```python
from build123d import *

# Parameters (mm, degrees)
BOSS_EXTRUDE1_DEPTH      = 2
BOSS_EXTRUDE1_DEPTH_BACK = 3
SKETCH1_R                = 16
SKETCH1_R_2              = 1.75
SKETCH1_R_3              = 1.25
SKETCH2_R                = 4.95
SKETCH2_R_2              = 2.95
BOSS_EXTRUDE3_DEPTH      = 3
SKETCH5_R                = 3.5
CUT_EXTRUDE2_DEPTH       = 4
SKETCH6_R                = 18
SKETCH6_R_2              = 16
BOSS_EXTRUDE4_DEPTH      = 5
CUT_EXTRUDE3_DEPTH       = 10
CUT_EXTRUDE3_DEPTH_BACK  = 3
SKETCH7_R                = 11
SKETCH8_R                = 5
CUT_EXTRUDE4_DEPTH       = 3


with BuildPart() as part:
    # Sketch1 → Boss-Extrude1 (new, two sides: drawn at the far end of the back side and taken through both)
    with BuildSketch(Plane(origin=(0, 0, 0), x_dir=(1, 0, 0), z_dir=(0, 1, 0)).offset(-BOSS_EXTRUDE1_DEPTH_BACK)):
        with Locations(Location((0, 0, 0), (0, 0, 270))):
            Circle(SKETCH1_R)
        with Locations(Location((0, 0, 0), (0, 0, 270))):
            Circle(SKETCH1_R_2, mode=Mode.SUBTRACT)
        with Locations(Location((-13.5, 0, 0), (0, 0, 270))):
            Circle(SKETCH1_R_3, mode=Mode.SUBTRACT)
        with Locations(Location((-4.171729424, 12.83926297, 0), (0, 0, 270))):
            Circle(SKETCH1_R_3, mode=Mode.SUBTRACT)
        with Locations(Location((10.921729424, 7.935100906, 0), (0, 0, 270))):
            Circle(SKETCH1_R_3, mode=Mode.SUBTRACT)
        with Locations(Location((10.921729424, -7.935100906, 0), (0, 0, 270))):
            Circle(SKETCH1_R_3, mode=Mode.SUBTRACT)
        with Locations(Location((-4.171729424, -12.83926297, 0), (0, 0, 270))):
            Circle(SKETCH1_R_3, mode=Mode.SUBTRACT)
    extrude(amount=BOSS_EXTRUDE1_DEPTH + BOSS_EXTRUDE1_DEPTH_BACK)

    # Sketch2 → Boss-Extrude3 (add)
    with BuildSketch(Plane(origin=(0, 2, 0), x_dir=(1, 0, 0), z_dir=(0, 1, 0))):
        with Locations(Location((0, 0, 0), (0, 0, 270))):
            Circle(SKETCH2_R)
        with Locations(Location((0, 0, 0), (0, 0, 270))):
            Circle(SKETCH2_R_2, mode=Mode.SUBTRACT)
    extrude(amount=BOSS_EXTRUDE3_DEPTH)

    # Sketch5 → Cut-Extrude2 (cut)
    with BuildSketch(Plane.XZ.offset(3)):
        with Locations(Location((0, 0, 0), (0, 0, 270))):
            Circle(SKETCH5_R)
    extrude(amount=-CUT_EXTRUDE2_DEPTH, mode=Mode.SUBTRACT)

    # Sketch6 → Boss-Extrude4 (add)
    with BuildSketch(Plane(origin=(0, 2, 0), x_dir=(1, 0, 0), z_dir=(0, 1, 0))):
        with Locations(Location((0, 0, 0), (0, 0, 270))):
            Circle(SKETCH6_R)
        Circle(SKETCH6_R_2, mode=Mode.SUBTRACT)
    extrude(amount=-BOSS_EXTRUDE4_DEPTH)

    # Sketch7 → Cut-Extrude3 (cut, two sides: drawn at the far end of the back side and taken through both)
    with BuildSketch(Plane(origin=(0, 2, 0), x_dir=(1, 0, 0), z_dir=(0, 1, 0)).offset(-CUT_EXTRUDE3_DEPTH_BACK)):
        with Locations(Location((0, 0, 0), (0, 0, 270))):
            Circle(SKETCH7_R)
    extrude(amount=CUT_EXTRUDE3_DEPTH + CUT_EXTRUDE3_DEPTH_BACK, mode=Mode.SUBTRACT)

    # Sketch8 → Cut-Extrude4 (cut)
    with BuildSketch(Plane(origin=(0, -1, 0), x_dir=(1, 0, 0), z_dir=(0, 1, 0))):
        with Locations(Location((0, 0, 0), (0, 0, 270))):
            Circle(SKETCH8_R)
    extrude(amount=-CUT_EXTRUDE4_DEPTH, mode=Mode.SUBTRACT)


solid = part.part
```
Model file for the job. Use its own axes, mm. A direction names the side the tool comes from. Coordinates: 2 decimals unless noted, no trailing zeros. Order: outer loops, then holes, each group sorted by start corner. A loop starts at its lowest first (then second) coordinate and runs counter-clockwise, first axis right, second up. Notation, with made-up numbers: (18.25, -2) -> (29.25, -2) arc R9 ccw to (29.25, 5) -> close; hole circle Ø11 at (35.25, -29.5). An arc over 180 degrees is marked (long way). Return JSON: item names as keys, results as strings.
Item 1: Slice it at B-B (z = 0). Write the cut outline in (x, y).
Model answer:
{"outline": "(-18, -3) -> (-14.75, -3) -> (-14.75, 2) -> (-18, 2) -> close; (-12.25, -3) -> (-5, -3) -> (-5, -1) -> (-11, -1) -> (-11, 2) -> (-12.25, 2) -> close; (5, -3) -> (18, -3) -> (18, 2) -> (11, 2) -> (11, -1) -> (5, -1) -> close"}
Item 2: Slice it at C-C (x = 10.5). Write the cut outline in (y, z).
Model answer:
{"outline": "(-3, -14.62) -> (2, -14.62) -> (2, -9.11) -> (-3, -9.11) -> close; (-3, -6.76) -> (2, -6.76) -> (2, -3.28) -> (-1, -3.28) -> (-1, 3.28) -> (2, 3.28) -> (2, 6.76) -> (-3, 6.76) -> close; (-3, 9.11) -> (2, 9.11) -> (2, 14.62) -> (-3, 14.62) -> close"}
Item 3: 3-axis set-ups, long thin cutter, end or side, ignore diameter. For faces 1 (the face through (-10.74, 0.48, -2.38)), 2 (the face through (10.161, -0.535, -8.927)): which of +Z, -Z, +X, -X, +Y, -Y reach the whole face in a straight line?
Model answer:
{"face 1": "+Y", "face 2": "+Y, -Y"}
Item 4: Mould opens along X. For faces 3 (the face through (10.161, -0.535, 6.943)), 4 (the face through (5.407, -0.465, 17.169)), 5 (the face through (-4.65, -0.535, 13.994)), 6 (the face through (8, 2, 8)) say: pulls with the +X half, pulls with the -X half, needs draft (parallel to the pull), parting line crosses it, or undercut.
Model answer:
{"face 3": "undercut", "face 4": "parting line crosses it", "face 5": "undercut", "face 6": "needs draft"}
Item 5: Slice it at D-D (y = 1). Write the cut outline in (x, z).
Model answer:
{"outline": "circle Ø36 at (0, 0); hole circle Ø2.5 at (-13.5, 0); hole circle Ø22 at (0, 0); hole circle Ø2.5 at (-4.17, -12.84); hole circle Ø2.5 at (-4.17, 12.84); hole circle Ø2.5 at (10.92, -7.94); hole circle Ø2.5 at (10.92, 7.94)"}
Item 6: Wall check: line 1 along X through (y, z) = (0.45, 0); line 2 along X through (y, z) = (0.45, -7); line 3 along Z through (x, y) = (12, -1.6). Give the ranges that are in metal, low to high. Write a range as from..to.
Model answer:
{"line 1": "x = -18..-14.75, -12.25..-11, 11..18", "line 2": "x = -16.58..-8.49, 8.49..10.09, 11.75..16.58", "line 3": "z = -13.42..-8.57, -7.3..7.3, 8.57..13.42"}
Item 7: Pin check, flat tips, straight feed: P1, Ø2, axis at x = -4.17, z = -12.84, coming from the +Y side; P2, Ø3, axis at y = -0.5, z = -7.5, coming from the +X side; P3, Ø2, axis at x = -7.5, y = -0.5, coming from the -Z side; P4, Ø2, axis at x = -8, y = 0.5, coming from the +Z side. Stop position of each tip, or through.
Model answer:
{"P1": "passes through", "P2": "stops at x = 16.97", "P3": "stops at z = -16.79", "P4": "stops at z = 16.58"}
Item 8: Slice it at A-A (x = 0). Write the cut outline in (y, z).
Model answer:
{"outline": "(-3, -18) -> (2, -18) -> (2, -11) -> (-1, -11) -> (-1, -5) -> (-3, -5) -> close; (-3, 5) -> (-1, 5) -> (-1, 11) -> (2, 11) -> (2, 18) -> (-3, 18) -> close"}
